Geometry: final body of the model. Coordinates: model frame, mm. A direction names the side the tool comes from. Give positions to 0.01 mm unless a question says otherwise; leave off trailing zeros. Order: outer loops, then holes, each group sorted by start corner. A loop starts at its lowest first (then second) coordinate and runs counter-clockwise, first axis right, second up. Notation, with made-up numbers: (57.5, 1.25) -> (108.5, 1.25) arc R30 cw to (108.5, 34.25) -> close; hole circle Ø2 at (39, 82). An arc over 180 degrees is marked (long way). Write item = value, one per line.
```python
from build123d import *

# Parameters (mm, degrees)
F0_R     = 1.5875
F1_DEPTH = 3.175


with BuildPart() as f1:
    # F0 (on Front) → F1 (new body)
    with BuildSketch(Plane.XZ):
        with BuildLine():
            Line((92.075, 0), (3.175, 0))
            ThreePointArc((3.175, 0), (0.929936, -0.929936), (0, -3.175))
            Line((0, -3.175), (0, -123.825))
            ThreePointArc((0, -123.825), (0.929936, -126.070064), (3.175, -127))
            Line((3.175, -127), (92.075, -127))
            ThreePointArc((92.075, -127), (94.320064, -126.070064), (95.25, -123.825))
            Line((95.25, -123.825), (95.25, -3.175))
            ThreePointArc((95.25, -3.175), (94.320064, -0.929936), (92.075, 0))
        make_face()
        with Locations((12.7, -107.95)):
            Circle(F0_R, mode=Mode.SUBTRACT)
        with Locations((47.625, -114.3)):
            Circle(F0_R, mode=Mode.SUBTRACT)
        with BuildLine():
            Line((25.4, -93.98), (69.85, -93.98))
            ThreePointArc((69.85, -93.98), (72.095064, -94.909936), (73.025, -97.155))
            Line((73.025, -97.155), (73.025, -106.045))
            ThreePointArc((73.025, -106.045), (72.095064, -108.290064), (69.85, -109.22))
            Line((69.85, -109.22), (25.4, -109.22))
            ThreePointArc((25.4, -109.22), (23.154936, -108.290064), (22.225, -106.045))
            Line((22.225, -106.045), (22.225, -97.155))
            ThreePointArc((22.225, -97.155), (23.154936, -94.909936), (25.4, -93.98))
        make_face(mode=Mode.SUBTRACT)
        with Locations((82.55, -107.95)):
            Circle(F0_R, mode=Mode.SUBTRACT)
        with Locations((47.625, -69.85)):
            Circle(F0_R, mode=Mode.SUBTRACT)
        with Locations((9.525, -46.954749)):
            Circle(F0_R, mode=Mode.SUBTRACT)
        with Locations((12.7, -10.16)):
            Circle(F0_R, mode=Mode.SUBTRACT)
        with BuildLine():
            ThreePointArc((22.225, -24.564049), (23.154936, -22.318984), (25.4, -21.389049))
            Line((25.4, -21.389049), (69.85, -21.389049))
            ThreePointArc((69.85, -21.389049), (72.095064, -22.318984), (73.025, -24.564049))
            Line((73.025, -24.564049), (73.025, -62.664049))
            ThreePointArc((73.025, -62.664049), (72.095064, -64.909113), (69.85, -65.839049))
            Line((69.85, -65.839049), (25.4, -65.839049))
            ThreePointArc((25.4, -65.839049), (23.154936, -64.909113), (22.225, -62.664049))
            Line((22.225, -62.664049), (22.225, -24.564049))
        make_face(mode=Mode.SUBTRACT)
        with Locations((85.725, -46.954749)):
            Circle(F0_R, mode=Mode.SUBTRACT)
        with Locations((82.55, -10.16)):
            Circle(F0_R, mode=Mode.SUBTRACT)
    extrude(amount=F1_DEPTH)


solid = f1.part
```
1) Line query: line 1 (Z direction, x = 53, y = -1); line 2 (Z direction, x = 12.7, y = -1.65); line 3 (X direction, y = -0.95, z = -36) (3 decimals). Output: solid intervals per line, ascending. Write a range as from..to.
Check sheet entries:
line_1 = -127..-109.22, -93.98..-65.84, -21.39..0
line_2 = -127..-109.54, -106.36..-11.75, -8.57..0
line_3 = 0..22.225, 73.025..95.25
2) Section query A-A (x = 82.55). Output: boundary loops of the cut face in (y, z) (1 decimal), plus the area to 3 significant figures.
Check sheet entries:
outline = (-3.2, -127) -> (0, -127) -> (0, -109.5) -> (-3.2, -109.5) -> close; (-3.2, -106.4) -> (0, -106.4) -> (0, -11.7) -> (-3.2, -11.7) -> close; (-3.2, -8.6) -> (0, -8.6) -> (0, 0) -> (-3.2, 0) -> close
area = 383 mm²
3) Mould query, pull axis Z, two halves, no side actions, for faces 1 (the face through (0.91, -1.57, -126.05)), 2 (the face through (47, -3.175, -77)), 3 (the face through (94.34, -1.57, -0.95)), 4 (the face through (23.13, -1.565, -94.935)). Classes: +Z half, -Z half, draft (parallel to the pull), parting line (faces both ways), or undercut.
Check sheet entries:
face_1 = -Z half
face_2 = draft
face_3 = +Z half
face_4 = undercut
4) Section query C-C (z = -10.16). Count the separate pieces of the cut face and the enclosed holes in it, plus the area to 3 significant figures.
Check sheet entries:
separate_pieces = 3
enclosed_holes = 0
area = 282 mm²
5) Reachability of faces 5 (the face through (94.3, -1.57, -126.09)), 6 (the face through (72.07, -1.565, -94.885)) from +Z, -Z, +X, -X, +Y, -Y: full face, straight path, thin tool, end or side. Return the list, or none.
Check sheet entries:
face_5 = -Z, +X, +Y, -Y
face_6 = +Y, -Y
